Here's how the part is built. I have some questions about the finished solid (model axes, mm). Give positions to 0.01 mm unless a question says otherwise; leave off trailing zeros. Loops run counter-clockwise (first coordinate to the right, second up) from the corner with the lowest first, then second, coordinate; pieces in that order, holes last.
Q1. Will these pins go through, and if not, where does the flat tip stop? P1, Ø1.5, axis at x = -1.5, z = 5.5, coming from the +Y side; P2, Ø4, axis at y = 1, z = 2.5, coming from the +X side; P3, Ø1.5, axis at y = 3, z = 7.5, coming from the +X side; P4, Ø4, axis at y = -3.5, z = 7.5, coming from the +X side.
Q2. If we section it at B-B (x = 3.5): Please give me the cut outline in (y, z), plus the area to 3 significant figures.
Q3. If we section it at A-A (z = 7.5): Please give me the cut outline in (x, y), plus the area to 3 significant figures.
Q4. I need wall thicknesses on line 1 (Y direction, x = 0, z = 7.75); line 2 (Y direction, x = 1.25, z = -1); line 3 (Z direction, x = -5.5, y = -2). Which ranges of each line are inside material? Lowest first, please.
Autodesk Inventor part; units mm, degrees
ref_plane "YZ Plane" through (0, 0, 0) normal (1, 0, 0) x (0, 1, 0)
ref_plane "XZ Plane" through (0, 0, 0) normal (0, 1, 0) x (-1, 0, 0)
ref_plane "XY Plane" through (0, 0, 0) normal (0, 0, 1) x (1, 0, 0)
sketch "Sketch1" plane through (0.3113, 7.3239, 0) normal (0, 0, -1) x (-1, 0, 0)
  circle A0 centre (0.3113, -7.3239) radius 6.5
  circle A1 centre (0.3113, -7.3239) radius 1.5
  dimension "d0" = 13
  dimension "d1" = 3
extrude "Extrusion1" add sketch "Sketch1" along normal blind 6 and the other way blind 10
ref_plane "Work Plane1" through (-5.7325, -3.064, 0) normal (-0.8819, -0.4714, 0) x (0.4714, -0.8819, 0)
sketch "Sketch2" plane through (-5.7325, -3.064, 0) normal (-0.8819, -0.4714, 0) x (0.4714, -0.8819, 0)
  circle A0 centre (0, -2) radius 2
  point P0 (0, 0)
  dimension "d6" = 4
  dimension "d7" = 2
extrude "Extrusion2" cut sketch "Sketch2" against normal blind 8
properties part number "gears_3mm_17TModded"
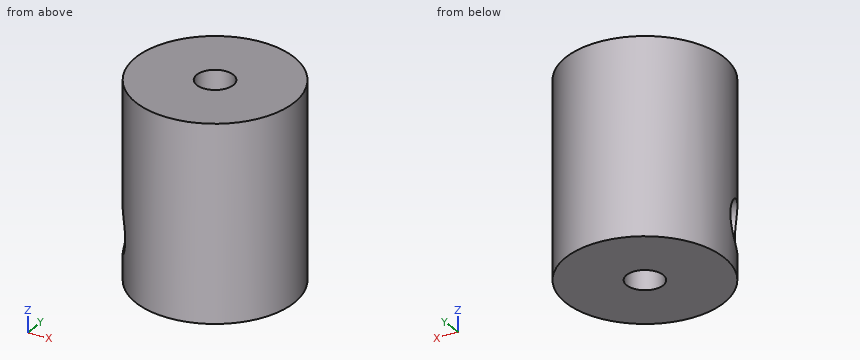
Check sheet entries:
1. P1: stops at y = 6.46
1. P2: stops at x = 6.5
1. P3: stops at x = 6.1
1. P4: stops at x = 6.32
2. outline: (-5.48, -6) - (5.48, -6) - (5.48, 10) - (-5.48, 10) - close
2. area: 175 mm2
3. outline: circle Ø13 at (0, 0); hole circle Ø3 at (0, 0)
3. area: 126 mm2
4. line 1: y = -6.5 to -1.5, 1.5 to 6.5
4. line 2: y = -6.38 to -1.3, 0.85 to 6.38
4. line 3: z = -6 to -3.82, -0.18 to 10
